from build123d import *

# Parameters (mm, degrees)
F0_W     = 50.8
F0_H     = 50.8
F0_R     = 12.7
F1_DEPTH = 50.8
F2_R     = 12.7
F3_DEPTH = 12.7
F4_W     = 25.4
F4_H     = 21.145677
F5_DEPTH = 12.7


with BuildPart() as f1:
    # F0 (on Front) → F1 (new body)
    with BuildSketch(Plane.XZ):
        with Locations((-10.655479, 25.4)):
            Rectangle(F0_W, F0_H)
        with Locations((-10.875792, 26.120912)):
            Circle(F0_R, mode=Mode.SUBTRACT)
    extrude(amount=F1_DEPTH)

    # F2 (on face) → F3 (join)
    with BuildSketch(Plane.XY.offset(50.8)):
        with Locations((-12.352031, -24.81534)):
            Circle(F2_R)
    extrude(amount=F3_DEPTH)

    # F4 (on face) → F5 (join)
    with BuildSketch(Plane(origin=(0, 0, 0), x_dir=(1, 0, 0), z_dir=(0, 0, -1))):
        with Locations((-12.7, 24.083575)):
            Rectangle(F4_W, F4_H)
    extrude(amount=F5_DEPTH)


solid = f1.part
For this review, take the finished solid that the model builds, in its own axes (mm). A direction names the side the tool comes from. Round coordinates to 2 decimals unless told otherwise and drop trailing zeros. Loops run counter-clockwise (first coordinate to the right, second up) from the corner with the lowest first, then second, coordinate; pieces in that order, holes last. Notation, with made-up numbers: (84.25, 21) - (107.25, 21) arc R16 cw to (107.25, 43) - close; hole circle Ø10 at (48, 16.5). An arc over 180 degrees is marked (long way). Use one line per item in the form item = value.
Item 1: Consider section B-B on x = -7.5. Write out the cut boundary in (y, z).
Answers:
outline = (-50.8, 0) - (-34.66, 0) - (-34.66, -12.7) - (-13.51, -12.7) - (-13.51, 0) - (0, 0) - (0, 13.88) - (-50.8, 13.88) - close; (-50.8, 38.36) - (0, 38.36) - (0, 50.8) - (-13.08, 50.8) - (-13.08, 63.5) - (-36.55, 63.5) - (-36.55, 50.8) - (-50.8, 50.8) - close
Item 2: Consider section A-A on z = 27.5. Write out the cut boundary in (x, y).
Answers:
outline = (-36.06, -50.8) - (-23.5, -50.8) - (-23.5, 0) - (-36.06, 0) - close; (1.75, -50.8) - (14.74, -50.8) - (14.74, 0) - (1.75, 0) - close
Item 3: For line 1 (X direction, y = -9, z = 19); line 2 (X direction, y = -30, z = 30); line 3 (Z direction, x = -27, y = -42.5), list the stretches that pass through material, from the lowest coordinate up.
Answers:
line_1 = -36.06 to -21.39, -0.36 to 14.74
line_2 = -36.06 to -22.97, 1.22 to 14.74
line_3 = 0 to 50.8
Item 4: Tool access review of faces 1 (the cylindrical face through (-15.105, -37.213, 57.061)), 2 (the flat face through (-13, -13.511, -6)), 3 (the flat face through (0, -24, -6)), 4 (the flat face through (-13, -34.656, -6)): name each direction out of +Z, -Z, +X, -X, +Y, -Y from which nothing blocks a thin tool from reaching the whole face with its end or side.
Answers:
face_1 = +Z
face_2 = -Z, +X, -X, +Y
face_3 = -Z, +X, +Y, -Y
face_4 = -Z, +X, -X, -Y
Item 5: Consider section C-C on y = -18. Write out the cut boundary in (x, z).
Answers:
outline = (-36.06, 0) - (-25.4, 0) - (-25.4, -12.7) - (0, -12.7) - (0, 0) - (14.74, 0) - (14.74, 50.8) - (-1.64, 50.8) - (-1.64, 63.5) - (-23.07, 63.5) - (-23.07, 50.8) - (-36.06, 50.8) - close; hole circle Ø25.4 at (-10.88, 26.12)
Item 6: Consider section D-D on x = -14.5. Write out the cut boundary in (y, z), then the cut area to 3 significant figures.
Answers:
outline = (-50.8, 0) - (-34.66, 0) - (-34.66, -12.7) - (-13.51, -12.7) - (-13.51, 0) - (0, 0) - (0, 13.95) - (-50.8, 13.95) - close; (-50.8, 38.29) - (0, 38.29) - (0, 50.8) - (-12.3, 50.8) - (-12.3, 63.5) - (-37.33, 63.5) - (-37.33, 50.8) - (-50.8, 50.8) - close
area = 1,930 mm^2
Item 7: Mouldability with a two-part tool opening along X and no side actions: class faces 5 (the flat face through (-25.4, -24, -6)), 6 (the flat face through (-17, -50.8, 14)), 7 (the cylindrical face through (-4, -25, 36.8)) as +X half, -X half, draft (parallel to the pull), parting line (faces both ways), or undercut.
Answers:
face_5 = -X half
face_6 = draft
face_7 = undercut
Item 8: Clearance check with flat-ended pins moving along their axes: P1, Ø4, axis at x = -16.5, z = -6.5, coming from the +Y side; P2, Ø4, axis at x = -17.5, z = -3.5, coming from the -Y side; P3, Ø4, axis at y = -22.5, z = -7, coming from the +X side. State where each tip first meets the part, or that it passes through.
Answers:
P1 = -13.51
P2 = -34.66
P3 = 0
